The model under review builds one solid part; all positions refer to its coordinate system, in mm. A direction names the side the tool comes from. Coordinates: 2 decimals unless noted, no trailing zeros. Put each result on its own line as item: value.
from build123d import *

# Parameters (mm, degrees)
F0_R            = 14.2875
F1_DEPTH        = 7.9375
F2_R            = 15.875
F3_DEPTH        = 6.35
F4_R            = 0.79375
F5_DEPTH        = 7.9375
F5_COPIES_COUNT = 4


# Not quite as in the source:
# - a pattern or mirror of a feature is missing from the dataset's text; its kind, count and spacing are read off the source's solid


with BuildPart() as f1:
    # F0 (on Top) → F1 (new body)
    with BuildSketch(Plane.XY):
        Polygon((19.05, 11.90625), (15.875, 11.90625), (15.875, 15.875), (11.90625, 15.875), (11.90625, 19.05), (-11.90625, 19.05), (-11.90625, 15.875), (-15.875, 15.875), (-15.875, 11.90625), (-19.05, 11.90625), (-19.05, -11.90625), (-15.875, -11.90625), (-15.875, -15.875), (-11.90625, -15.875), (-11.90625, -19.05), (11.90625, -19.05), (11.90625, -15.875), (15.875, -15.875), (15.875, -11.90625), (19.05, -11.90625), align=None)
        Circle(F0_R, mode=Mode.SUBTRACT)
    extrude(amount=F1_DEPTH)

    # F2 (on face) → F3 (cut)
    with BuildSketch(Plane.XY.offset(7.9375)):
        Circle(F2_R)
    extrude(amount=-F3_DEPTH, mode=Mode.SUBTRACT)

    # F4 (on face) → F5 (cut, through all)
    with BuildSketch(Plane.XY.offset(7.9375)):
        with Locations((11.90625, 15.875)):
            Circle(F4_R)
        with Locations((-11.90625, 15.875)):
            Circle(F4_R)
    f5 = extrude(amount=-F5_DEPTH, mode=Mode.SUBTRACT)

    # F5_copies: F5 ×4 about axis
    f5_copies_axis = Axis((0, 0, 0), (0, 0, 1))
    for i in range(1, F5_COPIES_COUNT):
        add(f5.rotate(f5_copies_axis, i * 360 / F5_COPIES_COUNT), mode=Mode.SUBTRACT)


solid = f1.part
Item 1: For faces 1 (the flat face through (-14, 15.875, 4)), 2 (the flat face through (15.875, 14, 4)), 3 (the flat face through (-11.906, -18, 4)), list the 3-axis set-ups (+Z, -Z, +X, -X, +Y, -Y) from which the entire face can be reached by the end or side of a thin tool; tool diameter is ignored.
Answers below:
face 1: +Z, -Z, -X, +Y
face 2: +Z, -Z, +X, +Y
face 3: +Z, -Z, -X, -Y
Item 2: For line 1 (X direction, y = 10.5, z = 6.25); line 2 (Y direction, x = 0, z = 4.75) (3 decimals); line 3 (Y direction, x = 0, z = 0.4), list the stretches that pass through material, from the lowest coordinate up. Write a range as from..to.
Answers below:
line 1: -19.05..-11.91, 11.91..19.05
line 2: -19.05..-15.875, 15.875..19.05
line 3: -19.05..-14.29, 14.29..19.05
Item 3: Mouldability with a two-part tool opening along X and no side actions: class faces 4 (the cylindrical face through (11.33, 15.33, 4.02)), 5 (the flat face through (14, -15.875, 4)), 6 (the flat face through (15.875, -14, 4)) as +X half, -X half, draft (parallel to the pull), parting line (faces both ways), or undercut.
Answers below:
face 4: undercut
face 5: draft
face 6: +X half
Item 4: For pin 1 Ø3.5 at (x, z) = (-14.5, 3.5) entering from +Y (3 decimals); pin 2 Ø1.2 at (y, z) = (-18, 2.5) entering from +X; pin 3 Ø1.3 at (x, y) = (-15.88, -11.91) entering from +Z; pin 4 Ø5 at (x, y) = (14.5, -2) entering from -Z, all flat-tipped, find the tip position at first contact; note any pin that passes through.
Answers below:
pin 1: y = 15.875
pin 2: x = 11.91
pin 3: through
pin 4: z = 0
